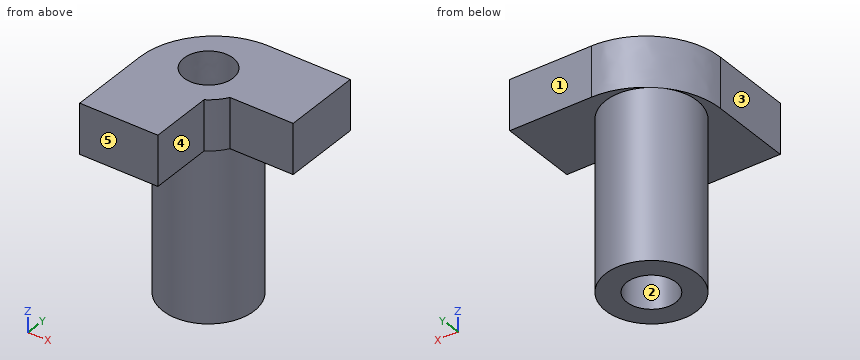
from build123d import *

# Parameters (mm, degrees)
SALIENTE_EXTRUIR1_DEPTH = 3.2
CROQUIS2_R              = 2.9227085
SALIENTE_EXTRUIR2_DEPTH = 10.8
CROQUIS3_R              = 1.571228252
CORTAR_EXTRUIR1_DEPTH   = 13.8
CORTAR_EXTRUIR2_DEPTH   = 13.8


with BuildPart() as part:
    # Model → Saliente-Extruir1 (new body)
    with BuildSketch(Plane.XY):
        with BuildLine():
            Line((-3.452848132, -1.30644903), (-3.452848132, -6.530212538))
            Line((-3.452848132, -6.530212538), (6.547151868, -6.530212538))
            Line((6.547151868, -6.530212538), (6.547151868, 3.469787462))
            Line((6.547151868, 3.469787462), (1.32338836, 3.469787462))
            add(Edge.make_bspline(
                [(-3.452848132, -1.30644903), (-3.452848132, 1.32052565), (-1.303487189, 3.469787462), (1.32338836, 3.469787462)],
                knots=[0.777777778, 0.777777778, 0.777777778, 0.777777778, 1, 1, 1, 1], degree=3))
        make_face()
        with BuildLine():
            add(Edge.make_bspline(
                [(0.016741068, 1.571228252), (-2.704706095, 1.571228252), (-1.343982514, -0.785614126), (0.016741068, -3.142456504), (1.377464649, -0.785614126), (2.73818823, 1.571228252), (0.016741068, 1.571228252)],
                knots=[0, 0, 0, 2.094395102, 2.094395102, 4.188790205, 4.188790205, 6.283185307, 6.283185307, 6.283185307], degree=2, weights=[1, 0.5, 1, 0.5, 1, 0.5, 1]))
        make_face(mode=Mode.SUBTRACT)
    extrude(amount=SALIENTE_EXTRUIR1_DEPTH)

    # Croquis2 → Saliente-Extruir2 (add)
    with BuildSketch(Plane(origin=(0, 0, 0), x_dir=(-1, 0, 0), z_dir=(0, 0, -1))):
        with Locations((-0.016741068, 0)):
            Circle(CROQUIS2_R)
    extrude(amount=SALIENTE_EXTRUIR2_DEPTH)

    # Croquis3 → Cortar-Extruir1 (cut)
    with BuildSketch(Plane.XY):
        with Locations((0.016741068, 0)):
            Circle(CROQUIS3_R)
    extrude(amount=-CORTAR_EXTRUIR1_DEPTH, mode=Mode.SUBTRACT)

    # Croquis4 → Cortar-Extruir2 (cut)
    with BuildSketch(Plane(origin=(0, 0, 0), x_dir=(-1, 0, 0), z_dir=(0, 0, -1))):
        with BuildLine():
            Line((-13.440411088, -13.370534454), (-1.547151868, -13.370534454))
            Line((-1.547151868, -13.370534454), (-1.547151868, -2.489993526))
            ThreePointArc((-1.547151868, -2.489993526), (-2.083490341, -2.066584722), (-2.506856439, -1.530212538))
            Line((-2.506856439, -1.530212538), (-13.440411088, -1.530212538))
            Line((-13.440411088, -1.530212538), (-13.440411088, -13.370534454))
        make_face()
    extrude(amount=-CORTAR_EXTRUIR2_DEPTH, mode=Mode.SUBTRACT)


solid = part.part
Part model, mm, in its own coordinate system. Face numbers are marked on the shaded views. A direction names the side the tool comes from. Round coordinates to 2 decimals unless told otherwise and drop trailing zeros. Write each loop counter-clockwise with the first axis right and the second up, starting at its lowest first coordinate (ties: lowest second). Pieces come first, ordered by that corner, then holes. Notation, with made-up numbers: M 11,41.5 L 70,41.5 A16 ccw 70,48.5 Z; hole C 50.5,42 d5. An arc over 180 degrees is marked long. Return JSON: item names as keys, results as strings. Group by question number.
(1) Which spindle directions (+Z, -Z, +X, -X, +Y, -Y) get a long thin tool onto all of the face, cutting with end or side? Do the marked faces 4 and 5. Say none if no direction does.
(2) Saw through at D-D on y = -5.25. Write the cut outline in (x, z).
(3) Drill centre lines: probe 1 along X at (y, z) = (0, -7); probe 2 along Y at (x, z) = (0.5, -7); probe 3 along Z at (x, y) = (2.5, 2.75). Where is each one in solid material? Low to high.
(4) Saw through at B-B on y = -2.75. Write the cut outline in (x, z).
(5) Saw through at A-A on z = -0.5. Write the cut outline in (x, y), then the cut area to 3 significant figures.
(6) Saw through at C-C on x = 4.75. Write the cut outline in (y, z).
(7) Pin check, flat tips, straight feed: pin 1 Ø6 at (x, z) = (0.5, -6) entering from -Y; pin 2 Ø1.5 at (x, y) = (0.5, -5.5) entering from -Z; pin 3 Ø3.5 at (x, z) = (4, 1) entering from -Y; pin 4 Ø2 at (x, y) = (4, -4.5) entering from -Z. Stop position of each tip, or through.
(8) Two-plate mould, pull along X, no slides. Class the marked faces 1, 2 and 3: +X half, -X half, draft (parallel to the pull), parting line (faces both ways), or undercut.
Returned:
{
 "1": {"face 4": "+Z, -Z, +X, -Y", "face 5": "+Z, -Z, +X, -X, -Y"},
 "2": {"outline": "M -3.45,0 L 1.55,0 L 1.55,3.2 L -3.45,3.2 Z"},
 "3": {"probe 1": "-2.91 to -1.55, 1.59 to 2.94", "probe 2": "-2.88 to -1.5, 1.5 to 2.88", "probe 3": "0 to 3.2"},
 "4": {"outline": "M -3.45,0 L -0.97,0 L -0.97,-10.8 L 1.01,-10.8 L 1.01,0 L 1.55,0 L 1.55,3.2 L -3.45,3.2 Z"},
 "5": {"outline": "C 0.02,0 d5.85; hole C 0.02,0 d3.14", "area": "19.1 mm²"},
 "6": {"outline": "M -1.53,0 L 3.47,0 L 3.47,3.2 L -1.53,3.2 Z"},
 "7": {"pin 1": "y = -2.92", "pin 2": "z = 0", "pin 3": "y = -1.89", "pin 4": "through"},
 "8": {"face 1": "draft", "face 2": "undercut", "face 3": "-X half"}
}
